```python
from build123d import *

# Parameters (mm, degrees)
SKETCH1_W               = 53.825
SKETCH1_H               = 38.5
MAIN_EXTRUDE_DEPTH      = 2.3
WALLS_DEPTH             = 35
SKETCH36_W              = 7
SKETCH36_H              = 2.3
SKETCH36_W_2            = 2.3
SKETCH36_H_2            = 7
PUZZLE_MAIN_WALLS_DEPTH = 3.175
SKETCH25_W              = 10.403042977
SKETCH25_H              = 6.605151166
WIRE_HOLE_DEPTH         = 3.3
SKETCH19_W              = 6.5
SKETCH19_H              = 12.025
SKETCH19_W_2            = 6
IR_MOUNT_DEPTH          = 7
MAGNET_MOUNT_HOLE_DEPTH = 51.83
SKETCH40_R              = 1.5
LED_SPACE_DEPTH         = 3
SKETCH42_W              = 7
SKETCH42_H              = 2.3
BOSS_EXTRUDE15_DEPTH    = 3.175
SKETCH44_W              = 6
SKETCH44_H              = 12.025
SKETCH44_W_2            = 6.5
BOSS_EXTRUDE16_DEPTH    = 6
SKETCH45_W              = 5
SKETCH45_H              = 5
IR_PLACEMENT_DEPTH      = 12.025
SKETCH47_R              = 2.5
CUT_EXTRUDE2_DEPTH      = 2
SKETCH48_W              = 7
SKETCH48_H              = 9
CUT_EXTRUDE3_DEPTH      = 15
BOSS_EXTRUDE17_DEPTH    = 3.175
SKETCH51_W              = 22.5
SKETCH51_H              = 10
BOSS_EXTRUDE18_DEPTH    = 4
BOSS_EXTRUDE19_DEPTH    = 6
SKETCH54_W              = 7
SKETCH54_H              = 2.3
CUT_EXTRUDE5_DEPTH      = 9.6


with BuildPart() as part:
    # Sketch1 → main extrude (new body)
    with BuildSketch(Plane(origin=(0, 0, 0), x_dir=(0, 0, -1), z_dir=(1, 0, 0))):
        with Locations((-26.9125, 21.443980352)):
            Rectangle(SKETCH1_W, SKETCH1_H)
    extrude(amount=MAIN_EXTRUDE_DEPTH)

    # Sketch3 → walls (add)
    with BuildSketch(Plane(origin=(2.3, 0, 0), x_dir=(0, 0, -1), z_dir=(1, 0, 0))):
        Polygon((-2.3, 38.393980352), (-2.3, 10.693980352), (-53.825, 10.693980352), (-53.825, 2.193980352), (0, 2.193980352), (0, 40.693980352), (-53.825, 40.693980352), (-53.825, 38.393980352), align=None)
    extrude(amount=WALLS_DEPTH)

    # Sketch36 → Puzzle (main walls) (add)
    with BuildSketch(Plane.XY.offset(53.825)):
        with Locations((11.5, 39.543980352)):
            Rectangle(SKETCH36_W, SKETCH36_H)
        with Locations((26.5, 39.543980352)):
            Rectangle(SKETCH36_W, SKETCH36_H)
        with Locations((1.15, 29.193980352)):
            Rectangle(SKETCH36_W_2, SKETCH36_H_2)
        with Locations((1.15, 14.193980352)):
            Rectangle(SKETCH36_W_2, SKETCH36_H_2)
    extrude(amount=PUZZLE_MAIN_WALLS_DEPTH)

    # Sketch25 → Wire Hole (cut, through all)
    with BuildSketch(Plane.XY.offset(2.3)):
        with Locations((7.501521489, 13.996555935)):
            Rectangle(SKETCH25_W, SKETCH25_H)
    extrude(amount=-WIRE_HOLE_DEPTH, mode=Mode.SUBTRACT)

    # Sketch19 → IR mount (add)
    with BuildSketch(Plane(origin=(0, 10.693980352, 0), x_dir=(1, 0, 0), z_dir=(0, 1, 0))):
        with Locations((34.05, -47.8125)):
            Rectangle(SKETCH19_W, SKETCH19_H)
        with Locations((5.3, -47.8125)):
            Rectangle(SKETCH19_W_2, SKETCH19_H)
    extrude(amount=IR_MOUNT_DEPTH)

    # Sketch24 → Magnet Mount Hole (cut)
    with BuildSketch(Plane.XY.offset(53.83)):
        Polygon((12.23, 2.193980352), (29.73, 2.193980352), (29.73, 5.693980352), (33.23, 5.693980352), (33.23, 8.693980352), (8.73, 8.693980352), (8.73, 5.693980352), (12.23, 5.693980352), align=None)
    extrude(amount=-MAGNET_MOUNT_HOLE_DEPTH, mode=Mode.SUBTRACT)

    # Sketch40 → LED Space (cut)
    with BuildSketch(Plane(origin=(0, 40.693980352, 0), x_dir=(1, 0, 0), z_dir=(0, 1, 0))):
        with Locations((19.3, -41.872631961)):
            Circle(SKETCH40_R)
    extrude(amount=-LED_SPACE_DEPTH, mode=Mode.SUBTRACT)

    # Sketch42 → Boss-Extrude15 (add)
    with BuildSketch(Plane(origin=(37.3, 0, 0), x_dir=(0, 0, -1), z_dir=(1, 0, 0))):
        with Locations((-42.325, 39.543980352)):
            Rectangle(SKETCH42_W, SKETCH42_H)
        with Locations((-14.5, 39.543980352)):
            Rectangle(SKETCH42_W, SKETCH42_H)
    extrude(amount=BOSS_EXTRUDE15_DEPTH)

    # Sketch44 → Boss-Extrude16 (add)
    with BuildSketch(Plane(origin=(0, 17.693980352, 0), x_dir=(1, 0, 0), z_dir=(0, 1, 0))):
        with Locations((5.3, -47.8125)):
            Rectangle(SKETCH44_W, SKETCH44_H)
        with Locations((34.05, -47.8125)):
            Rectangle(SKETCH44_W_2, SKETCH44_H)
    extrude(amount=BOSS_EXTRUDE16_DEPTH)

    # Sketch45 → IR placement (cut)
    with BuildSketch(Plane.XY.offset(53.825)):
        with Locations((33.3, 19.993980352)):
            Rectangle(SKETCH45_W, SKETCH45_H)
        with Locations((5.8, 19.993980352)):
            Rectangle(SKETCH45_W, SKETCH45_H)
    extrude(amount=-IR_PLACEMENT_DEPTH, mode=Mode.SUBTRACT)

    # Sketch47 → Cut-Extrude2 (cut)
    with BuildSketch(Plane(origin=(0, 0, 0), x_dir=(-1, 0, 0), z_dir=(0, 0, -1))):
        with Locations((-21.018982331, 5.262699137)):
            Circle(SKETCH47_R)
    extrude(amount=-CUT_EXTRUDE2_DEPTH, mode=Mode.SUBTRACT)

    # Sketch48 → Cut-Extrude3 (cut)
    with BuildSketch(Plane.XZ.offset(-2.193980352)):
        with Locations((3.5, 29.325)):
            Rectangle(SKETCH48_W, SKETCH48_H)
        with Locations((37.962462444, 29.325)):
            Rectangle(SKETCH48_W, SKETCH48_H)
    extrude(amount=-CUT_EXTRUDE3_DEPTH, mode=Mode.SUBTRACT)

    # Sketch50 → Boss-Extrude17 (add)
    with BuildSketch(Plane.XY.offset(53.825)):
        Polygon((37.3, 38.393980352), (2.3, 38.393980352), (2.3, 23.693980352), (8.3, 23.693980352), (8.3, 22.493980352), (3.3, 22.493980352), (3.3, 17.493980352), (8.3, 17.493980352), (8.3, 10.693980352), (30.8, 10.693980352), (30.8, 17.493980352), (35.8, 17.493980352), (35.8, 22.493980352), (30.8, 22.493980352), (30.8, 23.693980352), (37.3, 23.693980352), (37.3, 2.193980352), (29.73, 2.193980352), (29.73, 5.693980352), (33.23, 5.693980352), (33.23, 8.693980352), (8.73, 8.693980352), (8.73, 5.693980352), (12.23, 5.693980352), (12.23, 2.193980352), (0, 2.193980352), (0, 40.693980352), (37.3, 40.693980352), align=None)
    extrude(amount=BOSS_EXTRUDE17_DEPTH)

    # Sketch51 → Boss-Extrude18 (add)
    with BuildSketch(Plane(origin=(0, 10.693980352, 0), x_dir=(1, 0, 0), z_dir=(0, 1, 0))):
        with Locations((19.55, -52)):
            Rectangle(SKETCH51_W, SKETCH51_H)
    extrude(amount=BOSS_EXTRUDE18_DEPTH)

    # Sketch52 → Boss-Extrude19 (add)
    with BuildSketch(Plane(origin=(0, 10.693980352, 0), x_dir=(1, 0, 0), z_dir=(0, 1, 0))):
        Polygon((9.3, -47.4), (29.8, -47.4), (29.8, -57), (30.8, -57), (30.8, -47), (30.8, -45), (8.3, -45), (8.3, -47), (8.3, -57), (9.3, -57), align=None)
    extrude(amount=BOSS_EXTRUDE19_DEPTH)

    # Sketch54 → Cut-Extrude5 (cut)
    with BuildSketch(Plane.XY.offset(57)):
        with Locations((19.55, 39.543980352)):
            Rectangle(SKETCH54_W, SKETCH54_H)
        with Locations((19.55, 13.543980352)):
            Rectangle(SKETCH54_W, SKETCH54_H)
    extrude(amount=-CUT_EXTRUDE5_DEPTH, mode=Mode.SUBTRACT)


solid = part.part
```
Source: CAD feature listing. Evaluate the final solid. Frame: model axes, mm. A direction names the side the tool comes from. Coordinates: 2 decimals unless noted, no trailing zeros. Order: outer loops, then holes, each group sorted by start corner. A loop starts at its lowest first (then second) coordinate and runs counter-clockwise, first axis right, second up. Notation, with made-up numbers: M -40,34 L -12,34 A14 cw -12,40 Z; hole C -33.75,-25.5 d10. An arc over 180 degrees is marked long. Write each question's results on one line, items separated by ' | '. Start each with the question number.
1) Access query for faces 4 (the face through (20, 12.394, 52)), 5 (the face through (19.105, 39.56, 40.385)), 6 (the face through (3, 8, 24.825)), 7 (the face through (29.8, 16, 52)). Directions: +Z, -Z, +X, -X, +Y, -Y. A direction counts if a zero-diameter tool reaches every point of the face in a straight line with its end or side. Return the directions, or none.
2) Line query: line 1 (Y direction, x = 9.5, z = 52.5); line 2 (Y direction, x = 30, z = 42); line 3 (Z direction, x = 19.3, y = 39.55). Output: solid intervals per line, ascending. Write a range as from..to.
3) Draft query along Z for faces 1 (the face through (34, 16, 41.8)), 2 (the face through (1, 17.194, 29)), 3 (the face through (13, 14.694, 52)). Return one class per face: released by +Z, released by -Z, zero draft, split by the parting line, or undercut.
4) Section query D-D (z = 20). Return the cut outline in (x, y).
5) Contact query for flat-ended pins moving along their axis: pin 1 Ø5 at (y, z) = (25, 12) entering from +X; pin 2 Ø1.3 at (y, z) = (23, 47.5) entering from +X; pin 3 Ø1.8 at (x, y) = (39.5, 39.5) entering from -Z. Output: stop coordinate, or through.
6) Section query B-B (y = 7). Return the cut outline in (x, z) (3 decimals), plus the area to 3 significant figures.
7) Section query C-C (x = 19.3). Return the cut outline in (y, z).
8) Section query A-A (z = 30.5). Return the cut outline in (x, y).
Answers:
1) face 4: +Z, +Y | face 5: +Y | face 6: -X, -Y | face 7: +Z
2) line 1: y = 2.19..5.69, 8.69..14.69, 38.39..40.69 | line 2: y = 2.19..5.69, 8.69..10.69, 38.39..40.69 | line 3: z = 0..40.37, 43.37..47.4
3) face 1: undercut | face 2: undercut | face 3: zero draft
4) outline: M 0,2.19 L 12.23,2.19 L 12.23,5.69 L 8.73,5.69 L 8.73,8.69 L 33.23,8.69 L 33.23,5.69 L 29.73,5.69 L 29.73,2.19 L 37.3,2.19 L 37.3,10.69 L 2.3,10.69 L 2.3,38.39 L 37.3,38.39 L 37.3,40.69 L 0,40.69 Z
5) pin 1: stops at x = 2.3 | pin 2: stops at x = 37.3 | pin 3: stops at z = 11
6) outline: M 0,0 L 19.221,0 L 19.221,2 L 8.73,2 L 8.73,57 L 0,57 L 0,33.825 L 7,33.825 L 7,24.825 L 0,24.825 Z; M 22.817,0 L 37.3,0 L 37.3,24.825 L 34.462,24.825 L 34.462,33.825 L 37.3,33.825 L 37.3,57 L 33.23,57 L 33.23,2 L 22.817,2 Z | area: 683 mm^2
7) outline: M 2.19,0 L 3.45,0 L 3.45,2 L 2.19,2 Z; M 7.08,0 L 40.69,0 L 40.69,40.37 L 38.39,40.37 L 38.39,2.3 L 10.69,2.3 L 10.69,45 L 16.69,45 L 16.69,47.4 L 12.39,47.4 L 12.39,57 L 8.69,57 L 8.69,2 L 7.08,2 Z; M 38.39,43.37 L 40.69,43.37 L 40.69,47.4 L 38.39,47.4 Z
8) outline: M 0,17.19 L 2.3,17.19 L 2.3,38.39 L 37.3,38.39 L 37.3,40.69 L 0,40.69 Z; M 7,2.19 L 12.23,2.19 L 12.23,5.69 L 8.73,5.69 L 8.73,8.69 L 33.23,8.69 L 33.23,5.69 L 29.73,5.69 L 29.73,2.19 L 34.46,2.19 L 34.46,10.69 L 7,10.69 Z
